Geometry: final body of the model. Coordinates: model frame, mm. Face numbers are marked on the shaded views. A direction names the side the tool comes from. Round coordinates to 2 decimals unless told otherwise and drop trailing zeros. Write each loop counter-clockwise with the first axis right and the second up, starting at its lowest first coordinate (ties: lowest second). Pieces come first, ordered by that corner, then holes. Notation, with made-up numbers: (20, -4.5) - (75, -4.5) arc R35 ccw to (75, 31.5) - close; hole circle Ø1 at (26, -2.75). An arc over 180 degrees is marked (long way). Write each question's results on one line, items separated by ' | '.
from build123d import *

# Parameters (mm, degrees)
SKETCH_1_R      = 2
EXTRUDE_1_DEPTH = 20


with BuildPart() as part:
    # 草图1 → 凸台-拉伸1 (new body)
    with BuildSketch(Plane.XY):
        with BuildLine():
            Line((-21, 18), (-18, 21))
            Line((-18, 21), (-10, 21))
            Line((-10, 21), (-10, 11.180339887))
            ThreePointArc((-10, 11.180339887), (0, -15), (10, 11.180339887))
            Line((10, 11.180339887), (10, 21))
            Line((10, 21), (18, 21))
            Line((18, 21), (21, 18))
            Line((21, 18), (21, -18))
            Line((21, -18), (18, -21))
            Line((18, -21), (-18, -21))
            Line((-18, -21), (-21, -18))
            Line((-21, -18), (-21, 18))
        make_face()
        with Locations((15.5, 15.5)):
            Circle(SKETCH_1_R, mode=Mode.SUBTRACT)
        with Locations((15.5, -15.5)):
            Circle(SKETCH_1_R, mode=Mode.SUBTRACT)
        with Locations((-15.5, -15.5)):
            Circle(SKETCH_1_R, mode=Mode.SUBTRACT)
        with Locations((-15.5, 15.5)):
            Circle(SKETCH_1_R, mode=Mode.SUBTRACT)
    extrude(amount=EXTRUDE_1_DEPTH)


solid = part.part
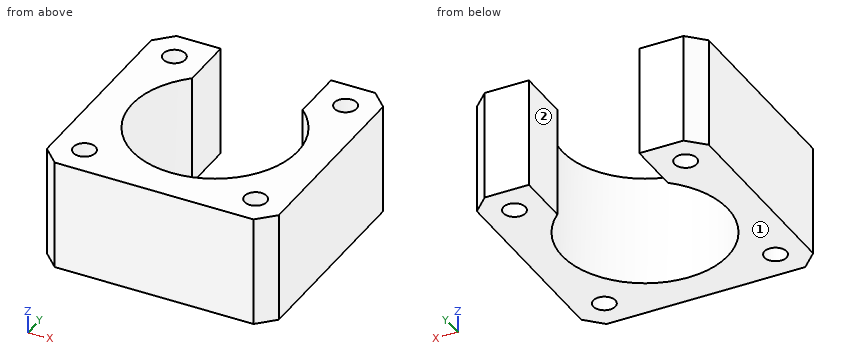
Q1. Section query B-B, the plane y = 15.5. Return loops of the section in (x, z).
Answer block:
outline: (-21, 0) - (-17.5, 0) - (-17.5, 20) - (-21, 20) - close; (-13.5, 0) - (-10, 0) - (-10, 20) - (-13.5, 20) - close; (10, 0) - (13.5, 0) - (13.5, 20) - (10, 20) - close; (17.5, 0) - (21, 0) - (21, 20) - (17.5, 20) - close
Q2. Section query D-D, the plane y = 5.5. Return loops of the section in (x, z).
Answer block:
outline: (-21, 0) - (-13.96, 0) - (-13.96, 20) - (-21, 20) - close; (13.96, 0) - (21, 0) - (21, 20) - (13.96, 20) - close
Q3. Ray query, line 1 along Y through (x, z) = (-15.5, 13); line 2 along X through (y, z) = (0, 11); line 3 along Y through (x, z) = (17, 15). Return the intervals inside material, ascending.
Answer block:
line 1: -21 to -17.5, -13.5 to 13.5, 17.5 to 21 | line 2: -21 to -15, 15 to 21 | line 3: -21 to -16.82, -14.18 to 14.18, 16.82 to 21
Q4. Section query A-A, the plane x = -12. Return loops of the section in (y, z).
Answer block:
outline: (-21, 0) - (-9, 0) - (-9, 20) - (-21, 20) - close; (9, 0) - (21, 0) - (21, 20) - (9, 20) - close
Q5. Section query C-C, the plane z = 2.25. Return loops of the section in (x, y), plus the area to 3 significant figures.
Answer block:
outline: (-21, -18) - (-18, -21) - (18, -21) - (21, -18) - (21, 18) - (18, 21) - (10, 21) - (10, 11.18) arc R15 cw (long way) to (-10, 11.18) - (-10, 21) - (-18, 21) - (-21, 18) - close; hole circle Ø4 at (-15.5, -15.5); hole circle Ø4 at (-15.5, 15.5); hole circle Ø4 at (15.5, -15.5); hole circle Ø4 at (15.5, 15.5) | area: 845 mm2
Q6. Access query for the marked faces 1 and 2. Directions: +Z, -Z, +X, -X, +Y, -Y. A direction counts if a zero-diameter tool reaches every point of the face in a straight line with its end or side. Return the directions, or none.
Answer block:
face 1: -Z, +X, -X, +Y, -Y | face 2: +Z, -Z, +Y
